Geometry: final body of the model. Coordinates: model frame, mm. A direction names the side the tool comes from. Coordinates: 2 decimals unless noted, no trailing zeros. Loops run counter-clockwise (first coordinate to the right, second up) from the corner with the lowest first, then second, coordinate; pieces in that order, holes last. Notation, with made-up numbers: (51, 35) - (109, 35) arc R5 ccw to (109, 42) - close; hole circle Ø8 at (27, 65.25). An arc over 180 degrees is marked (long way). Answer in a Markdown table with one row per item.
Autodesk Inventor part; units mm, degrees
ref_plane "YZ Plane" through (0, 0, 0) normal (1, 0, 0) x (0, 1, 0)
ref_plane "XZ Plane" through (0, 0, 0) normal (0, 1, 0) x (-1, 0, 0)
ref_plane "XY Plane" through (0, 0, 0) normal (0, 0, 1) x (1, 0, 0)
sketch "Sketch1" plane through (0, 0, 0) normal (0, 0, 1) x (1, 0, 0)
  line L0 (-105, -35) -> (105, -35)
  line L1 (105, -35) -> (105, 35)
  line L2 (105, 35) -> (-105, 35)
  line L3 (-105, 35) -> (-105, -35)
  line L4 (-105, -35) -> (105, 35) construction
  line L5 (105, -35) -> (-105, 35) construction
  point P0 (0, 0)
  dimension "d0" = 210
  dimension "d1" = 70
extrude "Extrusion1" add sketch "Sketch1" along normal blind 5
sketch "Sketch2" plane through (0, 0, 5) normal (0, 0, 1) x (1, 0, 0)
  line L0 (105, 35) -> (-105, 35)
  line L1 (-8.8, 35) -> (-8.8, 29.9)
  line L2 (-8.8, 29.9) -> (8.8, 29.9)
  line L3 (8.8, 29.9) -> (8.8, 35)
  line L4 (-43.8, 35) -> (-43.8, 29.9)
  line L5 (-43.8, 29.9) -> (-26.2, 29.9)
  line L6 (-26.2, 29.9) -> (-26.2, 35)
  line L7 (-78.8, 35) -> (-78.8, 29.9)
  line L8 (-78.8, 29.9) -> (-61.2, 29.9)
  line L9 (-61.2, 29.9) -> (-61.2, 35)
  line L10 (-113.8, 35) -> (-113.8, 29.9)
  line L11 (-113.8, 29.9) -> (-96.2, 29.9)
  line L12 (-96.2, 29.9) -> (-96.2, 35)
  line L13 (43.8, 29.9) -> (43.8, 35)
  line L14 (26.2, 29.9) -> (43.8, 29.9)
  line L15 (26.2, 35) -> (26.2, 29.9)
  line L16 (78.8, 29.9) -> (78.8, 35)
  line L17 (61.2, 29.9) -> (78.8, 29.9)
  line L18 (61.2, 35) -> (61.2, 29.9)
  line L19 (113.8, 29.9) -> (113.8, 35)
  line L20 (96.2, 29.9) -> (113.8, 29.9)
  line L21 (96.2, 35) -> (96.2, 29.9)
  line L22 (105, -35) -> (105, 35)
  line L23 (105, 35) -> (-105, 35)
  line L24 (-105, 35) -> (-105, -35)
  line L25 (-105, -35) -> (105, -35)
  line L26 (-99.9, 29.9) -> (-99.9, 11.6167)
  line L27 (-99.9, 11.6167) -> (-105, 11.6167)
  line L28 (99.9, 29.9) -> (99.9, 11.6167)
  line L29 (99.9, 11.6167) -> (105, 11.6167)
  point P0 (0, 0)
  point P1 (0, 35)
  point P2 (0, 29.9)
  point P3 (-8.8, 32.45)
  point P4 (8.8, 32.45)
  point P5 (-43.8, 32.45)
  point P6 (-35, 29.9)
  point P7 (-26.2, 32.45)
  point P8 (-35, 35)
  point P9 (-78.8, 32.45)
  point P10 (-70, 29.9)
  point P11 (-61.2, 32.45)
  point P12 (-70, 35)
  point P13 (-113.8, 32.45)
  point P14 (-105, 29.9)
  point P15 (-96.2, 32.45)
  point P16 (-105, 35)
  point P17 (26.2, 32.45)
  point P18 (35, 35)
  point P19 (35, 29.9)
  point P20 (43.8, 32.45)
  point P21 (61.2, 32.45)
  point P22 (70, 35)
  point P23 (70, 29.9)
  point P24 (78.8, 32.45)
  point P25 (96.2, 32.45)
  point P26 (105, 35)
  point P27 (105, 29.9)
  point P28 (113.8, 32.45)
  point P29 (105, 29.9)
  point P30 (-105, 35)
  point P31 (-105, 29.9)
  point P32 (-102.45, 11.6167)
  dimension "d4" = 5.1
  dimension "d5" = 17.6
  dimension "d6" = 210
  dimension "d24" = 35
  dimension "d31" = 35
  dimension "d36" = 70
  dimension "d37" = 23.3833
extrude "Extrusion2" cut sketch "Sketch2" against normal blind 5 contours L22 L20 L21 L0 | L22 L29 L28 L20 | L16 L17 L18 L0 | L13 L14 L15 L0 | L24 L11 L26 L27 | L3 L2 L1 L0 | L24 L0 L12 L11 | L6 L5 L4 L0 | L0 L9 L8 L7
sketch "Sketch4" plane through (0, 0, 0) normal (0, 0, -1) x (-1, 0, 0)
  line L0 (-85, -26.99) -> (0.6, -26.99)
  line L1 (0.6, -26.99) -> (0.6, 26.99)
  line L2 (0.6, 26.99) -> (-85, 26.99)
  line L3 (-85, 26.99) -> (-85, -26.99)
  line L4 (-85, -26.99) -> (0.6, 26.99) construction
  line L5 (0.6, -26.99) -> (-85, 26.99) construction
  line L6 (-105, -35) -> (-105, 35)
  line L7 (-85, 26.99) -> (0.0055, 26.99) construction
  line L8 (0.0055, 26.99) -> (0.0055, -27.0274) construction
  line L9 (0.0055, -27.0274) -> (-85, -27.0274) construction
  line L10 (-85, -27.0274) -> (-85, 26.99) construction
  point P0 (0, 0)
  point P1 (-42.2, 0)
  point P2 (-105, 29.9)
  dimension "d16" = 53.98
  dimension "d17" = 85.6
  dimension "d18" = 20
extrude "Extrusion4" cut sketch "Sketch4" against normal blind 0.5
sketch "Sketch3" plane through (0, 0, 0) normal (0, 0, -1) x (-1, 0, 0)
  line L0 (8.6, 25) -> (2.6, 25) construction
  line L1 (2.6, 25) -> (2.6, -25)
  line L2 (2.6, -25) -> (8.6, -25) construction
  line L3 (8.6, -25) -> (8.6, 25)
  line L4 (8.6, 25) -> (2.6, -25) construction
  line L5 (2.6, 25) -> (8.6, -25) construction
  arc A0 (2.6, -25) -> (8.6, -25) centre (5.6, -25) ccw
  arc A1 (8.6, 25) -> (2.6, 25) centre (5.6, 25) ccw
  line L6 (0.6, 26.99) -> (0.6, -26.99)
  line L7 (-85, 26.99) -> (0.6, 26.99)
  line L8 (-42.2, 26.99) -> (-42.2, -26.99)
  line L9 (0.6, -26.99) -> (-85, -26.99)
  line L10 (-93, 25) -> (-87, 25) construction
  line L11 (-87, 25) -> (-87, -25)
  line L12 (-87, -25) -> (-93, -25) construction
  line L13 (-93, -25) -> (-93, 25)
  line L14 (-93, 25) -> (-87, -25) construction
  line L15 (-87, 25) -> (-93, -25) construction
  arc A2 (-93, -25) -> (-87, -25) centre (-90, -25) ccw
  arc A3 (-87, 25) -> (-93, 25) centre (-90, 25) ccw
  point P0 (0, 0)
  point P1 (5.6, 0)
  point P2 (-90, 0)
  dimension "d12" = 6
  dimension "d13" = 50
  dimension "d21" = 5
extrude "Extrusion3" cut sketch "Sketch3" against normal blind 5 contours A1 L3 A0 L1 | L11 A2 L13 A3
mirror "Mirror2" about plane through (0, 0, 0) normal (0, 1, 0) of "Extrusion2"
sketch "Sketch5" plane through (0, 0, 0.5) normal (0, 0, -1) x (-1, 0, 0)
  line L0 (-85, 26.99) -> (0.0055, 26.99) construction
  line L1 (0.0055, 26.99) -> (0.0055, -27.0274) construction
  line L2 (0.0055, -27.0274) -> (-85, -27.0274) construction
  line L3 (-85, -27.0274) -> (-85, 26.99) construction
  point P0 (0, 0)
equation "\"d24\" = 0.166667 * d6"
properties part number "FloorPlate" material "MDF Medium Density Fiberboard"
(1) Cut plane D-D on x = 90. Output: boundary loops of the cut face in (y, z).
Verdict:
| item | result |
|---|---|
| outline | (-35, 0) - (-28, 0) - (-28, 5) - (-35, 5) - close; (28, 0) - (35, 0) - (35, 5) - (28, 5) - close |
(2) Cut plane B-B on y = -1.5. Output: boundary loops of the cut face in (x, z).
Verdict:
| item | result |
|---|---|
| outline | (-105, 0) - (-8.6, 0) - (-8.6, 5) - (-105, 5) - close; (-2.6, 0) - (-0.6, 0) - (-0.6, 0.5) - (85, 0.5) - (85, 0) - (87, 0) - (87, 5) - (-2.6, 5) - close; (93, 0) - (105, 0) - (105, 5) - (93, 5) - close |
(3) Ray query, probe 1 along X at (y, z) = (16.5, 2.5); probe 2 along X at (y, z) = (32.5, 4.4); probe 3 along X at (y, z) = (11.5, 2.1). Return the intervals inside material, ascending.
Verdict:
| item | result |
|---|---|
| probe 1 | x = -99.9 to -8.6, -2.6 to 87, 93 to 99.9 |
| probe 2 | x = -96.2 to -78.8, -61.2 to -43.8, -26.2 to -8.8, 8.8 to 26.2, 43.8 to 61.2, 78.8 to 96.2 |
| probe 3 | x = -105 to -8.6, -2.6 to 87, 93 to 105 |
(4) Access query for faces 4 (the face through (90, -28, 2)), 5 (the face through (8.8, -32, 3)), 6 (the face through (26.2, 32, 3)), 7 (the face through (96.2, 32, 3)), 8 (the face through (99.9, -21, 3)). Directions: +Z, -Z, +X, -X, +Y, -Y. A direction counts if a zero-diameter tool reaches every point of the face in a straight line with its end or side. Return the directions, or none.
Verdict:
| item | result |
|---|---|
| face 4 | +Z, -Z |
| face 5 | +Z, -Z, -Y |
| face 6 | +Z, -Z, +Y |
| face 7 | +Z, -Z, +X, +Y |
| face 8 | +Z, -Z, +X, -Y |
(5) Cut plane C-C on z = 1.6. State how many separate pieces and enclosed holes the cut face has, then the cut area to 3 significant figures.
Verdict:
| item | result |
|---|---|
| separate pieces | 1 |
| enclosed holes | 2 |
| area | 12,600 mm² |
(6) Cut plane A-A on x = -5.6. Output: boundary loops of the cut face in (y, z), then the cut area to 3 significant figures.
Verdict:
| item | result |
|---|---|
| outline | (-29.9, 0) - (-28, 0) - (-28, 5) - (-29.9, 5) - close; (28, 0) - (29.9, 0) - (29.9, 5) - (28, 5) - close |
| area | 19.0 mm² |
(7) First-contact query: pin 1 Ø1.5 at (x, z) = (69.5, 2.5) entering from -Y; pin 2 Ø2.5 at (y, z) = (33, 2) entering from +X; pin 3 Ø2.5 at (y, z) = (32.5, 3) entering from -X. Flat tips, straight axial feed; report the tip coordinate or a pass-through.
Verdict:
| item | result |
|---|---|
| pin 1 | stops at y = -29.9 |
| pin 2 | stops at x = 96.2 |
| pin 3 | stops at x = -96.2 |
(8) Pull-direction query (Y, two-part tool) for faces 1 (the face through (93, 0, 2)), 2 (the face through (52, -35, 2)), 3 (the face through (-78.8, 32, 3)); classes: pulls with the +Y half, pulls with the -Y half, needs draft (parallel to the pull), parting line crosses it, or undercut.
Verdict:
| item | result |
|---|---|
| face 1 | undercut |
| face 2 | pulls with the -Y half |
| face 3 | needs draft |
